The drawing under review shows one solid part. Ordinate dimensions are in mm from its lowest x, y, z. Coordinates: 2 decimals unless noted, no trailing zeros. Loops run counter-clockwise (first coordinate to the right, second up) from the corner with the lowest first, then second, coordinate; pieces in that order, holes last. Notation, with made-up numbers: (17.5, 71) -> (24.5, 71) arc R8 ccw to (24.5, 85) -> close; hole circle Ø10 at (-19.5, -16.75). An arc over 180 degrees is marked (long way). Use a Markdown table: item, result.
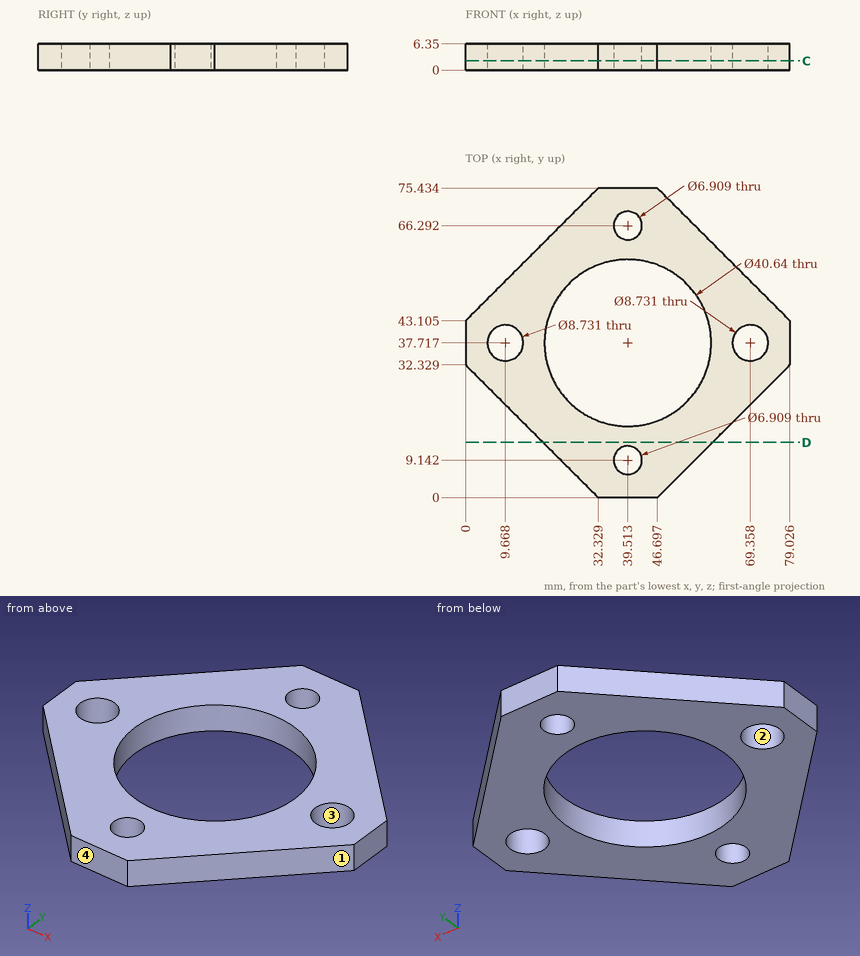
(1) Mouldability with a two-part tool opening along X and no side actions: class the marked faces 1, 2, 3 and 4 as pulls with the +X half, pulls with the -X half, needs draft (parallel to the pull), parting line crosses it, or undercut.
Found:
| item | result |
|---|---|
| face 1 | pulls with the +X half |
| face 2 | undercut |
| face 3 | undercut |
| face 4 | needs draft |
(2) For line 1 along X through (y, z) = (36, 1.5) (1 decimal); line 2 along Y through (x, z) = (45, 5.5) (1 decimal); line 3 along X through (y, z) = (23, 5.75) (1 decimal), list the stretches that pass through material, from the lowest coordinate up.
Found:
| item | result |
|---|---|
| line 1 | x = 0 to 5.7, 13.7 to 19.3, 59.8 to 65.3, 73.4 to 79 |
| line 2 | y = 0 to 18.2, 57.3 to 75.4 |
| line 3 | x = 9.3 to 25.5, 53.5 to 69.7 |
(3) For pin 1 Ø8 at (x, y) = (39.51, 9.14) entering from +Z; pin 2 Ø1.5 at (x, y) = (45, 21) entering from -Z, all flat-tipped, find the tip position at first contact; note any pin that passes through.
Found:
| item | result |
|---|---|
| pin 1 | stops at z = 6.35 |
| pin 2 | passes through |
(4) Take a section at D-D on y = 13.5. Write out the cut boundary in (x, z), plus the area to 3 significant figures.
Found:
| item | result |
|---|---|
| outline | (18.83, 0) -> (60.2, 0) -> (60.2, 6.35) -> (18.83, 6.35) -> close |
| area | 263 mm^2 |
(5) Take a section at C-C on z = 2.25. Write out the cut boundary in (x, y) (1 decimal), plus the area to 3 significant figures.
Found:
| item | result |
|---|---|
| outline | (0, 32.3) -> (32.3, 0) -> (46.7, 0) -> (79, 32.3) -> (79, 43.1) -> (46.7, 75.4) -> (32.3, 75.4) -> (0, 43.1) -> close; hole circle Ø8.7 at (9.7, 37.7); hole circle Ø40.6 at (39.5, 37.7); hole circle Ø6.9 at (39.5, 9.1); hole circle Ø6.9 at (39.5, 66.3); hole circle Ø8.7 at (69.4, 37.7) |
| area | 2,380 mm^2 |
